Job drawing, mm, ordinate dimensions from the low corner. One solid piece. A direction names the side the tool comes from. Round coordinates to 2 decimals unless told otherwise and drop trailing zeros. Loops run counter-clockwise (first coordinate to the right, second up) from the corner with the lowest first, then second, coordinate; pieces in that order, holes last. Notation, with made-up numbers: M 85,57 L 95,57 A14 cw 95,65 Z; hole C 17.25,12 d9. An arc over 180 degrees is marked long. Use one line per item in the form item = value.
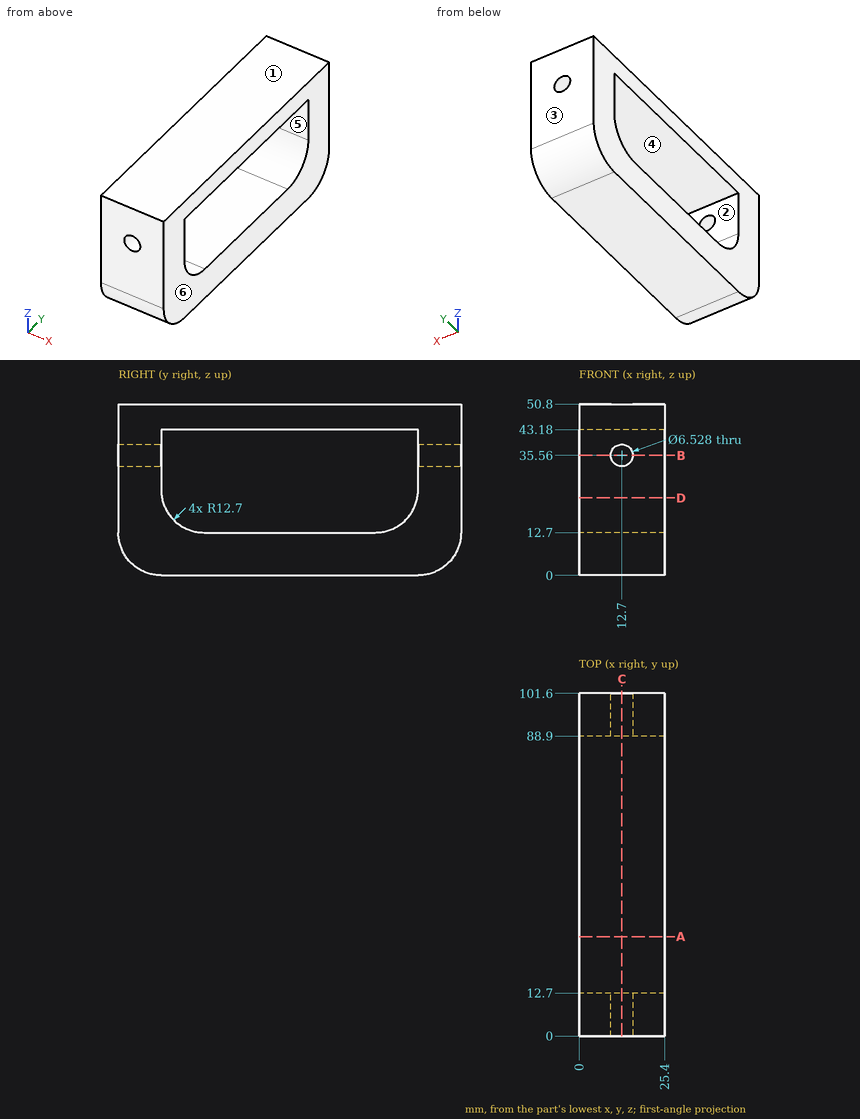
1. Cut at A-A on y = 29.5. Write the cut outline in (x, z), and give its area (3 significant figures).
Completed:
outline = M 0,0 L 25.4,0 L 25.4,12.7 L 0,12.7 Z; M 0,43.18 L 25.4,43.18 L 25.4,50.8 L 0,50.8 Z
area = 516 mm2
2. Drop flat-ended pins along their axis: P1, Ø2, axis at x = 17, z = 18.5, coming from the -Y side; P2, Ø1.5, axis at x = 10, y = 11.5, coming from the -Z side. Give the stop position or say it passes through.
Completed:
P1 = 0
P2 = 0.01
3. Tool access for the marked faces 1 and 2: list every direction of +Z, -Z, +X, -X, +Y, -Y with a clear straight run to the whole face (end or side of a thin tool).
Completed:
face_1 = +Z, +X, -X, +Y, -Y
face_2 = +X, -X
4. Cut at C-C on x = 12.7. Write the cut outline in (y, z).
Completed:
outline = M 0,12.7 A12.7 ccw 12.7,0 L 88.9,0 A12.7 ccw 101.6,12.7 L 101.6,32.3 L 88.9,32.3 L 88.9,25.4 A12.7 cw 76.2,12.7 L 25.4,12.7 A12.7 cw 12.7,25.4 L 12.7,32.3 L 0,32.3 Z; M 0,38.82 L 12.7,38.82 L 12.7,43.18 L 88.9,43.18 L 88.9,38.82 L 101.6,38.82 L 101.6,50.8 L 0,50.8 Z
5. Cut at B-B on z = 35.56. Write the cut outline in (x, y), and give its area (3 significant figures).
Completed:
outline = M 0,0 L 9.44,0 L 9.44,12.7 L 0,12.7 Z; M 0,88.9 L 9.44,88.9 L 9.44,101.6 L 0,101.6 Z; M 15.96,0 L 25.4,0 L 25.4,12.7 L 15.96,12.7 Z; M 15.96,88.9 L 25.4,88.9 L 25.4,101.6 L 15.96,101.6 Z
area = 479 mm2
6. Probe line 1 along X through (y, z) = (5.5, 35.56); line 2 along Z through (x, y) = (12.75, 70.5); line 3 along Y through (x, z) = (18.25, 37.5). List the from-to ranges inside material, lowest first. Write a range as from..to.
Completed:
line_1 = 0..9.44, 15.96..25.4
line_2 = 0..12.7, 43.18..50.8
line_3 = 0..12.7, 88.9..101.6
7. Pull direction Y, two halves, no side cores. Call the marked faces 3, 4, 5 and 6: +Y half, -Y half, draft (parallel to the pull), parting line (faces both ways), or undercut.
Completed:
face_3 = +Y half
face_4 = undercut
face_5 = undercut
face_6 = draft
8. Cut at D-D on z = 23. Write the cut outline in (x, y).
Completed:
outline = M 0,0 L 25.4,0 L 25.4,12.93 L 0,12.93 Z; M 0,88.67 L 25.4,88.67 L 25.4,101.6 L 0,101.6 Z
